from build123d import *

# Parameters (mm, degrees)
F1_DEPTH = 63.5
F2_DEPTH = 25.4
F0_W     = 19.693976
F0_H     = 19.05
F3_DEPTH = 25.4
F4_DEPTH = 7.9375


with BuildPart() as f1:
    # F0 (on Front) → F1 (new body, symmetric)
    with BuildSketch(Plane.XZ):
        Polygon((-41.275, 9.525), (-41.275, -9.525), (41.275, -9.525), (41.275, 9.525), (22.225, 9.525), align=None)
    extrude(amount=F1_DEPTH, both=True)

    # F0 (on Front) → F2 (join, symmetric)
    with BuildSketch(Plane.XZ):
        with BuildLine():
            Line((22.225, 9.525), (41.275, 9.525))
            Line((41.275, 9.525), (41.275, 27.0002))
            ThreePointArc((41.275, 27.0002), (45.92468, 38.22552), (57.15, 42.8752))
            Line((57.15, 42.8752), (60.325, 42.8752))
            Line((60.325, 42.8752), (60.325, 61.9252))
            add(Edge.make_bspline(
                [(50.017181, 61.189065), (53.471327, 61.494815), (56.914684, 61.73877), (60.325, 61.9252)],
                knots=[106.078682, 106.078682, 106.078682, 106.078682, 114.316845, 114.316845, 114.316845, 114.316845], degree=3))
            ThreePointArc((50.017181, 61.189065), (30.049545, 49.030201), (22.225, 27.0002))
            Line((22.225, 27.0002), (22.225, 9.525))
        make_face()
    extrude(amount=F2_DEPTH, both=True)

    # F0 (on Front) → F3 (join, symmetric)
    with BuildSketch(Plane.XZ):
        with Locations((70.171988, 52.4002)):
            Rectangle(F0_W, F0_H)
    extrude(amount=F3_DEPTH, both=True)

    # F0 (on Front) → F4 (join, symmetric)
    with BuildSketch(Plane.XZ):
        with BuildLine():
            add(Edge.make_bspline(
                [(-41.275, 9.525), (-40.72633, 43.06928), (5.539875, 57.25208), (50.017181, 61.189065)],
                knots=[0, 0, 0, 0, 106.078682, 106.078682, 106.078682, 106.078682], degree=3))
            Line((-41.275, 9.525), (22.225, 9.525))
            Line((22.225, 9.525), (22.225, 27.0002))
            ThreePointArc((22.225, 27.0002), (30.049545, 49.030201), (50.017181, 61.189065))
        make_face()
    extrude(amount=F4_DEPTH, both=True)


solid = f1.part
Geometry: final body of the model. Coordinates: model frame, mm. A direction names the side the tool comes from. Give positions to 0.01 mm unless a question says otherwise; leave off trailing zeros. Loops run counter-clockwise (first coordinate to the right, second up) from the corner with the lowest first, then second, coordinate; pieces in that order, holes last. Notation, with made-up numbers: M 13,42 L 29,42 A22 ccw 29,75 Z; hole C 27.5,61 d8. An arc over 180 degrees is marked long. Put each result on its own line as item: value.
1) Reachability of faces 1 (the flat face through (44, 25.4, 42)), 2 (the cylindrical face through (30.261, -16.791, 49.288)), 3 (the flat face through (68, 0, 42.875)), 4 (the flat face through (-5, 7.938, 30)) from +Z, -Z, +X, -X, +Y, -Y: full face, straight path, thin tool, end or side. Return the list, or none.
Computed values:
face 1: +Z, +X, -X, +Y
face 2: +Z, -X, -Y
face 3: -Z, +X, +Y, -Y
face 4: +Z, -X, +Y
2) First-contact query: P1, Ø14, axis at y = -18.5, z = 21.5, coming from the -X side (3 decimals); P2, Ø4, axis at x = 16, y = 12, coming from the +Z side (3 decimals); P3, Ø11, axis at y = -7.5, z = 3, coming from the +X side (3 decimals). Flat tips, straight axial feed; report the tip coordinate or a pass-through.
Computed values:
P1: stops at x = 22.225
P2: stops at z = 9.525
P3: stops at x = 41.275
3) Material intervals for L1, parallel to Y at x = 66.5, z = 46; L2, parallel to Z at x = -36, y = -15 (3 decimals); L3, parallel to Y at x = 23, z = 53, sorted ascending. Write a range as from..to.
Computed values:
L1: y = -25.4..25.4
L2: z = -9.525..9.525
L3: y = -7.94..7.94
4) Cut plane B-B, the plane y = 30.5. Return the cut outline in (x, z) (3 decimals), plus the area to 3 significant figures.
Computed values:
outline: M -41.275,-9.525 L 41.275,-9.525 L 41.275,9.525 L -41.275,9.525 Z
area: 1,570 mm^2
5) Cut plane A-A, the plane x = 65.5. Return the cut outline in (y, z), plus the area to 3 significant figures.
Computed values:
outline: M -25.4,42.88 L 25.4,42.88 L 25.4,61.93 L -25.4,61.93 Z
area: 968 mm^2
